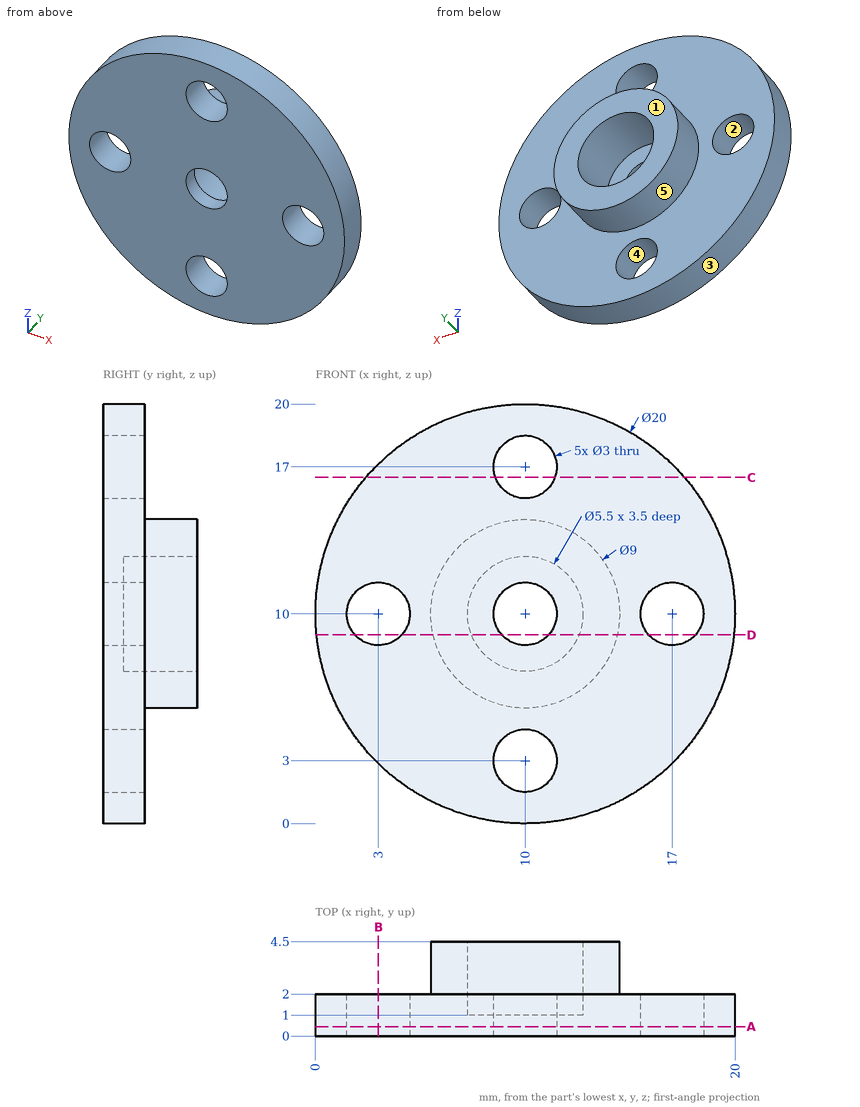
Geometry check sheet. Reference: drawing and pictorial views, mm from the part's lowest x, y, z. A direction names the side the tool comes from. Round coordinates to 2 decimals unless told otherwise and drop trailing zeros. Order: outer loops, then holes, each group sorted by start corner. A loop starts at its lowest first (then second) coordinate and runs counter-clockwise, first axis right, second up. Notation, with made-up numbers: M 64,86 L 80,86 A30 ccw 80,116 Z; hole C -11.5,4.25 d6. An arc over 180 degrees is marked long. Answer in a Markdown table with one row per item.
(1) Draft check along X on the marked faces 1, 2 and 3. Enter one of: released by +X, released by -X, zero draft, split by the parting line, or undercut.
Responses:
| item | result |
|---|---|
| face 1 | zero draft |
| face 2 | undercut |
| face 3 | split by the parting line |
(2) Scan lines: probe 1 along X at (y, z) = (1.15, 10); probe 2 along Z at (x, y) = (10, 0.65). Record each from-to range of solid material in increasing order. Write a range as from..to.
Responses:
| item | result |
|---|---|
| probe 1 | x = 0..1.5, 4.5..7.25, 12.75..15.5, 18.5..20 |
| probe 2 | z = 0..1.5, 4.5..8.5, 11.5..15.5, 18.5..20 |
(3) Go/stop test with flat-tipped pins: P1, Ø1.5, axis at x = 11, z = 8.5, coming from the +Y side; P2, Ø2, axis at x = 18, y = 2, coming from the -Z side. Record where each tip stops, or that it passes through.
Responses:
| item | result |
|---|---|
| P1 | stops at y = 1 |
| P2 | stops at z = 2.86 |
(4) Sectioned sample at C-C, the plane z = 16.5. Record the cut outline in (x, y), and give its area (3 significant figures).
Responses:
| item | result |
|---|---|
| outline | M 2.4,0 L 8.59,0 L 8.59,2 L 2.4,2 Z; M 11.41,0 L 17.6,0 L 17.6,2 L 11.41,2 Z |
| area | 24.7 mm² |
(5) Sectioned sample at A-A, the plane y = 0.45. Record the cut outline in (x, z), and give its area (3 significant figures).
Responses:
| item | result |
|---|---|
| outline | C 10,10 d20; hole C 3,10 d3; hole C 10,3 d3; hole C 10,10 d3; hole C 10,17 d3; hole C 17,10 d3 |
| area | 279 mm² |
(6) Sectioned sample at B-B, the plane x = 3. Record the cut outline in (y, z).
Responses:
| item | result |
|---|---|
| outline | M 0,2.86 L 2,2.86 L 2,8.5 L 0,8.5 Z; M 0,11.5 L 2,11.5 L 2,17.14 L 0,17.14 Z |
(7) Sectioned sample at D-D, the plane z = 9. Record the cut outline in (x, y), and give its area (3 significant figures).
Responses:
| item | result |
|---|---|
| outline | M 0.05,0 L 1.88,0 L 1.88,2 L 0.05,2 Z; M 4.12,0 L 8.88,0 L 8.88,1 L 7.44,1 L 7.44,4.5 L 5.61,4.5 L 5.61,2 L 4.12,2 Z; M 11.12,0 L 15.88,0 L 15.88,2 L 14.39,2 L 14.39,4.5 L 12.56,4.5 L 12.56,1 L 11.12,1 Z; M 18.12,0 L 19.95,0 L 19.95,2 L 18.12,2 Z |
| area | 32.6 mm² |
(8) Tool access check on the marked faces 4 and 5. Record the directions out of +Z, -Z, +X, -X, +Y, -Y that give a thin tool (end or side, any length) a straight path to the whole face; none if there is none.
Responses:
| item | result |
|---|---|
| face 4 | +Y, -Y |
| face 5 | +Y |
